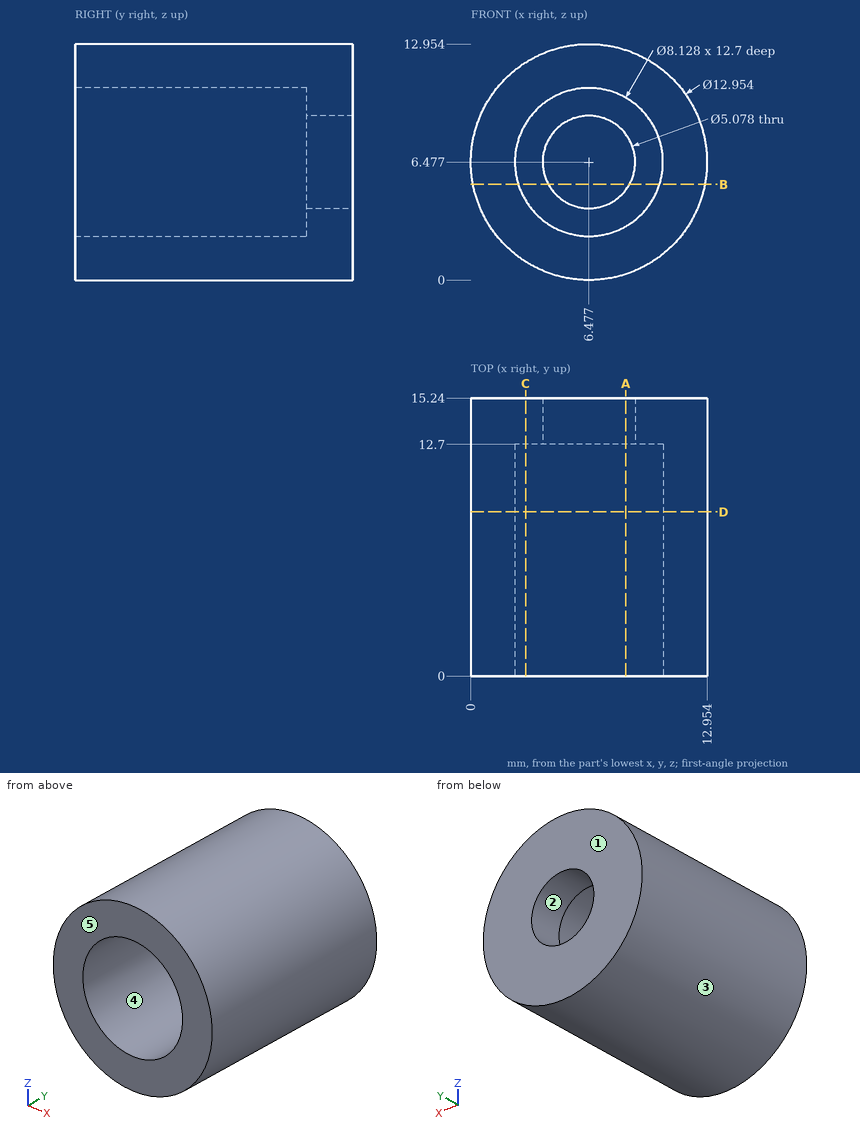
The drawing under review shows one solid part. Ordinate dimensions are in mm from its lowest x, y, z. A direction names the side the tool comes from. Round coordinates to 2 decimals unless told otherwise and drop trailing zeros. Loops run counter-clockwise (first coordinate to the right, second up) from the corner with the lowest first, then second, coordinate; pieces in that order, holes last. Notation, with made-up numbers: (35.5, -37) - (68.5, -37) arc R5 ccw to (68.5, -32) - close; hole circle Ø10 at (84.25, 73). An arc over 180 degrees is marked (long way). Use a Markdown table: item, result. Add a question column.
Q1. Add section B-B (z = 5.25). State the section outline as (x, y) points.
Q2. Insertion check: pin 1 Ø4 at (x, y) = (7, 11.5) entering from -Z; pin 2 Ø2 at (y, z) = (5.5, 3) entering from +X; pin 3 Ø4 at (x, z) = (5, 6) entering from -Y; pin 4 Ø2 at (x, y) = (10, 2.5) entering from -Z. Each pin has a flat end and moves straight along its axis. Give the tip position at first contact, or say it passes through.
Q3. Add section A-A (x = 8.5). State the section outline as (y, z) points.
Q4. For probe 1 along Z at (x, y) = (6.5, 3.25); probe 2 along Z at (x, y) = (8.75, 14); probe 3 along X at (y, z) = (9.5, 4.5) (3 decimals), list the stretches that pass through material, from the lowest coordinate up.
Q5. Machinability: for the marked faces 4 and 5, which of the approach directions +Z, -Z, +X, -X, +Y, -Y give a long, thin tool a straight path to every point of the face, cutting with its end or side? Answer none if there is none.
Q6. Add section C-C (x = 3). State the section outline as (y, z) points.
Q7. The part is to be moulded in two halves that separate along X. For the marked faces 1, 2 and 3, say which applies: pulls with the +X half, pulls with the -X half, needs draft (parallel to the pull), parting line crosses it, or undercut.
Q8. Add section D-D (y = 9). State the section outline as (x, z) points.
Worked answers:
| question | item | result |
|---|---|---|
| 1 | outline | (0.12, 0) - (2.6, 0) - (2.6, 12.7) - (4.25, 12.7) - (4.25, 15.24) - (0.12, 15.24) - close; (8.7, 12.7) - (10.35, 12.7) - (10.35, 0) - (12.84, 0) - (12.84, 15.24) - (8.7, 15.24) - close |
| 2 | pin 1 | z = 0 |
| 2 | pin 2 | x = 12.46 |
| 2 | pin 3 | y = 12.7 |
| 2 | pin 4 | z = 0.51 |
| 3 | outline | (0, 0.32) - (15.24, 0.32) - (15.24, 4.94) - (12.7, 4.94) - (12.7, 2.95) - (0, 2.95) - close; (0, 10) - (12.7, 10) - (12.7, 8.01) - (15.24, 8.01) - (15.24, 12.63) - (0, 12.63) - close |
| 4 | probe 1 | 0 to 2.41, 10.54 to 12.95 |
| 4 | probe 2 | 0.41 to 5.35, 7.61 to 12.54 |
| 4 | probe 3 | 0.309 to 2.926, 10.028 to 12.645 |
| 5 | face 4 | -Y |
| 5 | face 5 | +Z, -Z, +X, -X, -Y |
| 6 | outline | (0, 1.01) - (15.24, 1.01) - (15.24, 11.94) - (0, 11.94) - (0, 8.58) - (12.7, 8.58) - (12.7, 4.37) - (0, 4.37) - close |
| 7 | face 1 | needs draft |
| 7 | face 2 | undercut |
| 7 | face 3 | parting line crosses it |
| 8 | outline | circle Ø12.95 at (6.48, 6.48); hole circle Ø8.13 at (6.48, 6.48) |
